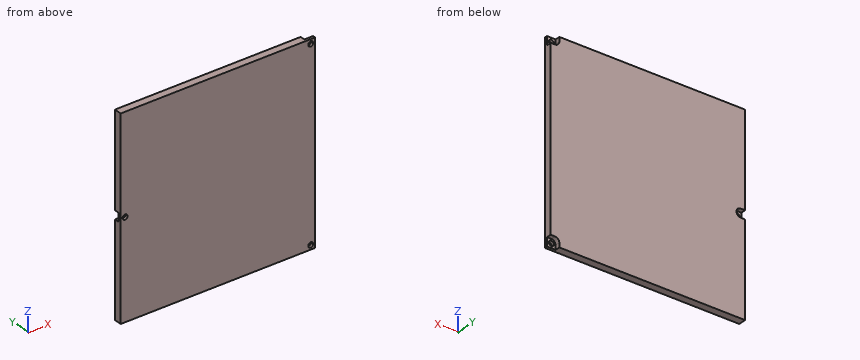
```python
from build123d import *

# Parameters (mm, degrees)
SKETCH1_W           = 203.2
SKETCH1_H           = 203.2
BOSS_EXTRUDE1_DEPTH = 7.9375
HOLES_REACH         = 9.938
SKETCH3_R           = 2.60985
SKETCH4_R           = 2.60985
COUNTERS_DEPTH      = 5.08


with BuildPart() as part:
    # Sketch1 → Boss-Extrude1 (new body)
    with BuildSketch(Plane(origin=(0, 0, 0), x_dir=(1, 0, 0), z_dir=(0, 1, 0))):
        with Locations((101.6, 101.6)):
            Rectangle(SKETCH1_W, SKETCH1_H)
    extrude(amount=BOSS_EXTRUDE1_DEPTH)

    # Sketch3 → holes (cut, up to next)
    with BuildSketch(Plane(origin=(0, 7.9375, 0), x_dir=(1, 0, 0), z_dir=(0, 1, 0)), mode=Mode.PRIVATE) as holes_sk1:
        with Locations((4.572, 101.6)):
            Circle(SKETCH3_R)
    holes_tool1 = extrude(holes_sk1.sketch, amount=-HOLES_REACH, mode=Mode.PRIVATE) & part.part
    add(holes_tool1.solids().sort_by_distance((4.572, 7.9375, -101.6))[0], mode=Mode.SUBTRACT)
    # Sketch3 → holes (cut, up to next)
    with BuildSketch(Plane(origin=(0, 7.9375, 0), x_dir=(1, 0, 0), z_dir=(0, 1, 0)), mode=Mode.PRIVATE) as holes_sk2:
        with Locations((198.628, 198.628)):
            Circle(SKETCH3_R)
    holes_tool2 = extrude(holes_sk2.sketch, amount=-HOLES_REACH, mode=Mode.PRIVATE) & part.part
    add(holes_tool2.solids().sort_by_distance((198.628, 7.9375, -198.628))[0], mode=Mode.SUBTRACT)
    # Sketch3 → holes (cut, up to next)
    with BuildSketch(Plane(origin=(0, 7.9375, 0), x_dir=(1, 0, 0), z_dir=(0, 1, 0)), mode=Mode.PRIVATE) as holes_sk3:
        with Locations((198.628, 4.572)):
            Circle(SKETCH3_R)
    holes_tool3 = extrude(holes_sk3.sketch, amount=-HOLES_REACH, mode=Mode.PRIVATE) & part.part
    add(holes_tool3.solids().sort_by_distance((198.628, 7.9375, -4.572))[0], mode=Mode.SUBTRACT)

    # Sketch4 → counters (cut)
    with BuildSketch(Plane(origin=(0, 7.9375, 0), x_dir=(1, 0, 0), z_dir=(0, 1, 0))):
        with BuildLine():
            Line((4.572, 106.0196), (0, 106.0196))
            Line((0, 106.0196), (0, 97.1804))
            Line((0, 97.1804), (4.572, 97.1804))
            ThreePointArc((4.572, 97.1804), (8.9916, 101.6), (4.572, 106.0196))
        make_face()
        with Locations((4.572, 101.6)):
            Circle(SKETCH4_R, mode=Mode.SUBTRACT)
        with BuildLine():
            Line((194.2084, 198.628), (194.2084, 203.2))
            Line((194.2084, 203.2), (203.2, 203.2))
            Line((203.2, 203.2), (203.2, 194.2084))
            Line((203.2, 194.2084), (198.628, 194.2084))
            ThreePointArc((198.628, 194.2084), (195.50287087, 195.50287087), (194.2084, 198.628))
        make_face()
        with Locations((198.628, 198.628)):
            Circle(SKETCH4_R, mode=Mode.SUBTRACT)
        with BuildLine():
            Line((194.2084, 4.572), (194.2084, 0))
            Line((194.2084, 0), (203.2, 0))
            Line((203.2, 0), (203.2, 8.9916))
            Line((203.2, 8.9916), (198.628, 8.9916))
            ThreePointArc((198.628, 8.9916), (195.50287087, 7.69712913), (194.2084, 4.572))
        make_face()
        with Locations((198.628, 4.572)):
            Circle(SKETCH4_R, mode=Mode.SUBTRACT)
    extrude(amount=-COUNTERS_DEPTH, mode=Mode.SUBTRACT)


solid = part.part
```
The listing builds one solid part. Answer for the finished solid, in the listing's coordinates (mm). Round coordinates to 2 decimals unless told otherwise and drop trailing zeros. Loops run counter-clockwise (first coordinate to the right, second up) from the corner with the lowest first, then second, coordinate; pieces in that order, holes last. Notation, with made-up numbers: (38, -27) -> (78, -27) arc R24 ccw to (78, 10) -> close; hole circle Ø4 at (21.25, 72). An arc over 180 degrees is marked (long way). Use one line per item in the form item = value.
1. The part is cut by section A-A on z = -101.6. Determine the outline of the cut face in (x, y), and give its area (3 significant figures).
Answer key:
outline = (0, 0) -> (1.96, 0) -> (1.96, 2.86) -> (0, 2.86) -> close; (7.18, 0) -> (203.2, 0) -> (203.2, 7.94) -> (8.99, 7.94) -> (8.99, 2.86) -> (7.18, 2.86) -> close
area = 1,550 mm²
2. Find the intervals of material crossed by probe 1 along X at (y, z) = (1.6, -101.6), in increasing order. Write a range as [from, to].
Answer key:
probe_1 = [0, 1.96], [7.18, 203.2]
3. Flat-ended cylindrical pins translate along their axes: pin 1 Ø6 at (x, z) = (198.628, -4.572) entering from +Y; pin 2 Ø3.5 at (x, y) = (202, 6) entering from +Z. Find the tip coordinate at first contact, or state that the pin passes through.
Answer key:
pin_1 = 2.86
pin_2 = -8.99
